Work out the finished part from the listing and answer in its coordinate system (mm). Face numbers are marked on the shaded views. A direction names the side the tool comes from. Coordinates: 2 decimals unless noted, no trailing zeros. Loops run counter-clockwise (first coordinate to the right, second up) from the corner with the lowest first, then second, coordinate; pieces in that order, holes last.
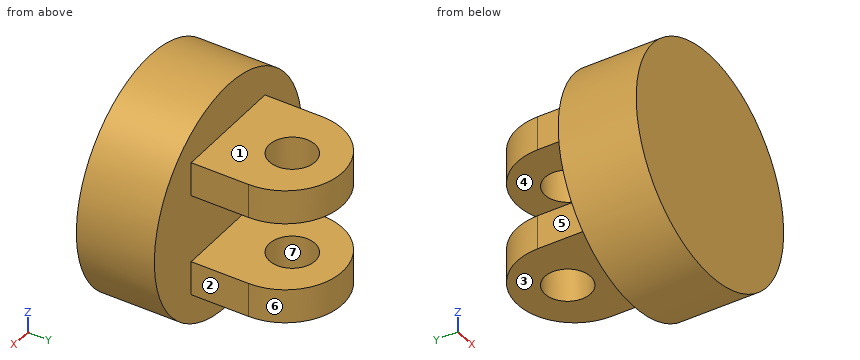
```python
from build123d import *

# Parameters (mm, degrees)
CROQUIS1_R              = 50
SALIENTE_EXTRUIR1_DEPTH = 34
CROQUIS2_W              = 50
CROQUIS2_H              = 15
SALIENTE_EXTRUIR2_DEPTH = 50
CROQUIS4_R              = 10
CORTAR_EXTRUIR1_DEPTH   = 60
REDONDEO1_RADIUS        = 25
REDONDEO1_LENGTH        = 15
REDONDEO2_RADIUS        = 25
REDONDEO2_LENGTH        = 15


with BuildPart() as part:
    # Croquis1 → Saliente-Extruir1 (new body)
    with BuildSketch(Plane(origin=(0, 0, 0), x_dir=(1, 0, 0), z_dir=(0, 1, 0))):
        with Locations(Location((0, 0, 0), (0, 0, 270))):
            Circle(CROQUIS1_R)
    extrude(amount=SALIENTE_EXTRUIR1_DEPTH)

    # Croquis2 → Saliente-Extruir2 (add)
    with BuildSketch(Plane(origin=(0, 34, 0), x_dir=(1, 0, 0), z_dir=(0, 1, 0))):
        with Locations((0, 22.5)):
            Rectangle(CROQUIS2_W, CROQUIS2_H)
        with Locations((0, -22.5)):
            Rectangle(CROQUIS2_W, CROQUIS2_H)
    extrude(amount=SALIENTE_EXTRUIR2_DEPTH)

    # Croquis4 → Cortar-Extruir1 (cut)
    with BuildSketch(Plane(origin=(0, 0, -30), x_dir=(-1, 0, 0), z_dir=(0, 0, -1))):
        with Locations((0, 62)):
            Circle(CROQUIS4_R)
    extrude(amount=-CORTAR_EXTRUIR1_DEPTH, mode=Mode.SUBTRACT)

    # Redondeo1: full round fillet: the end face becomes a half cylinder, R = half its width
    redondeo1_face = Plane((0, 84, -22.5), x_dir=(0, 0, 1), z_dir=(0, 1, 0))  # on the end face: x along it, z out of the body
    redondeo1_slab = redondeo1_face.offset(-REDONDEO1_RADIUS / 2) * Box(REDONDEO1_LENGTH, 2 * REDONDEO1_RADIUS, REDONDEO1_RADIUS, mode=Mode.PRIVATE)  # the body's end, R deep
    redondeo1_round = Plane((0, 59, -22.5), x_dir=(0, 1, 0), z_dir=(0, 0, 1)) * Cylinder(REDONDEO1_RADIUS, REDONDEO1_LENGTH, mode=Mode.PRIVATE)  # its axis R under the face
    add(redondeo1_slab - redondeo1_round, mode=Mode.SUBTRACT)

    # Redondeo2: full round fillet: the end face becomes a half cylinder, R = half its width
    redondeo2_face = Plane((0, 84, 22.5), x_dir=(0, 0, 1), z_dir=(0, 1, 0))  # on the end face: x along it, z out of the body
    redondeo2_slab = redondeo2_face.offset(-REDONDEO2_RADIUS / 2) * Box(REDONDEO2_LENGTH, 2 * REDONDEO2_RADIUS, REDONDEO2_RADIUS, mode=Mode.PRIVATE)  # the body's end, R deep
    redondeo2_round = Plane((0, 59, 22.5), x_dir=(0, 1, 0), z_dir=(0, 0, 1)) * Cylinder(REDONDEO2_RADIUS, REDONDEO2_LENGTH, mode=Mode.PRIVATE)  # its axis R under the face
    add(redondeo2_slab - redondeo2_round, mode=Mode.SUBTRACT)


solid = part.part
```
1. Straight lines are drawn through the part: probe 1 along Z at (x, y) = (-12, 63); probe 2 along Y at (x, z) = (0, 23); probe 3 along Y at (x, z) = (-35.5, -12). For each, find the intervals that lie inside material, in ascending order.
2. Determine the mould class of the marked faces 4, 5, 6 and 7 for opening direction X: released by +X, released by -X, zero draft, split by the parting line, or undercut.
3. Each of these flat-tipped pins is pushed along its axis until it touches: P1, Ø1.5, axis at x = -38.5, z = -27.5, coming from the +Y side; P2, Ø4.5, axis at y = 42, z = -26, coming from the +X side; P3, Ø15, axis at x = 4, y = 60, coming from the +Z side. Where does it stop, or does it pass through?
4. For the marked faces 1, 2 and 3, determine the directions among +Z, -Z, +X, -X, +Y, -Y from which every point of the face is accessible in a straight line to the end or side of a thin tool.
5. A cutting plane is placed at D-D, the plane z = -16.5. Give the vertices of the cut face in (x, y), then the cut area to 3 significant figures.
6. A cutting plane is placed at C-C, the plane y = 42. Give the vertices of the cut face in (x, z), then the cut area to 3 significant figures.
7. A cutting plane is placed at A-A, the plane y = 56. Give the vertices of the cut face in (x, z).
8. A cutting plane is placed at B-B, the plane x = 0. Give the vertices of the cut face in (y, z), then the cut area to 3 significant figures.
Answers below:
1. probe 1: z = -30 to -15, 15 to 30
1. probe 2: y = 0 to 52, 72 to 84
1. probe 3: y = 0 to 34
2. face 4: zero draft
2. face 5: released by -X
2. face 6: split by the parting line
2. face 7: undercut
3. P1: stops at y = 34
3. P2: stops at x = 25
3. P3: stops at z = 30
4. face 1: +Z, +X, -X, +Y
4. face 2: +Z, -Z, +X, +Y
4. face 3: -Z, +X, -X, +Y
5. outline: (-47.2, 0) - (47.2, 0) - (47.2, 34) - (25, 34) - (25, 59) arc R25 ccw to (-25, 59) - (-25, 34) - (-47.2, 34) - close; hole circle Ø20 at (0, 62)
5. area: 5,130 mm2
6. outline: (-25, -30) - (25, -30) - (25, -15) - (-25, -15) - close; (-25, 15) - (25, 15) - (25, 30) - (-25, 30) - close
6. area: 1,500 mm2
7. outline: (-25, -30) - (-8, -30) - (-8, -15) - (-25, -15) - close; (-25, 15) - (-8, 15) - (-8, 30) - (-25, 30) - close; (8, -30) - (25, -30) - (25, -15) - (8, -15) - close; (8, 15) - (25, 15) - (25, 30) - (8, 30) - close
8. outline: (0, -50) - (34, -50) - (34, -30) - (52, -30) - (52, -15) - (34, -15) - (34, 15) - (52, 15) - (52, 30) - (34, 30) - (34, 50) - (0, 50) - close; (72, -30) - (84, -30) - (84, -15) - (72, -15) - close; (72, 15) - (84, 15) - (84, 30) - (72, 30) - close
8. area: 4,300 mm2
